from build123d import *

# Parameters (mm, degrees)
SKETCH1_W           = 50
SKETCH1_H           = 15
SKETCH1_R           = 1.5
SKETCH1_R_2         = 5
BOSS_EXTRUDE1_DEPTH = 2.5
SKETCH2_R           = 6
CUT_EXTRUDE1_DEPTH  = 1000
SKETCH5_W           = 20
SKETCH5_H           = 15
BOSS_EXTRUDE2_DEPTH = 15
SKETCH2_5_R         = 6
CUT_EXTRUDE2_DEPTH  = 15
FILLET1_R           = 5
SKETCH6_R           = 1.25
CUT_EXTRUDE3_DEPTH  = 15


with BuildPart() as part:
    # Sketch1 → Boss-Extrude1 (new, symmetric)
    with BuildSketch(Plane(origin=(0, 0, 0), x_dir=(0, 0, -1), z_dir=(1, 0, 0))):
        with Locations((25, 7.5)):
            Rectangle(SKETCH1_W, SKETCH1_H)
        with Locations((10, 7.5)):
            Circle(SKETCH1_R, mode=Mode.SUBTRACT)
        with Locations((17.5, 7.5)):
            Circle(SKETCH1_R_2, mode=Mode.SUBTRACT)
        with Locations((25, 7.5)):
            Circle(SKETCH1_R, mode=Mode.SUBTRACT)
    extrude(amount=BOSS_EXTRUDE1_DEPTH, both=True)

    # Sketch2 → Cut-Extrude1 (cut)
    with BuildSketch(Plane(origin=(0, 15, 0), x_dir=(1, 0, 0), z_dir=(0, 1, 0))):
        with Locations((7.5, 42.75390625)):
            Circle(SKETCH2_R)
    extrude(amount=-CUT_EXTRUDE1_DEPTH, mode=Mode.SUBTRACT)

    # Sketch5 → Boss-Extrude2 (add)
    with BuildSketch(Plane(origin=(0, 15, 0), x_dir=(1, 0, 0), z_dir=(0, 1, 0))):
        with Locations((7.5, 42.5)):
            Rectangle(SKETCH5_W, SKETCH5_H)
    extrude(amount=-BOSS_EXTRUDE2_DEPTH)

    # Sketch2_5 → Cut-Extrude2 (cut)
    with BuildSketch(Plane(origin=(0, 15, 0), x_dir=(1, 0, 0), z_dir=(0, 1, 0))):
        with Locations(Location((7.5, 42.75390625, 0), (0, 0, 270))):
            Circle(SKETCH2_5_R)
    extrude(amount=-CUT_EXTRUDE2_DEPTH, mode=Mode.SUBTRACT)

    # Fillet1
    fillet1_edges = [part.edges().sort_by_distance(p)[0] for p in [
        (17.5, 7.5, -35),
        (17.5, 7.5, -50),
    ]]
    fillet(fillet1_edges, radius=FILLET1_R)

    # Sketch6 → Cut-Extrude3 (cut)
    with BuildSketch(Plane(origin=(17.5, 0, 0), x_dir=(0, 0, -1), z_dir=(1, 0, 0))):
        with Locations((42.5, 7.5)):
            Circle(SKETCH6_R)
    extrude(amount=-CUT_EXTRUDE3_DEPTH, mode=Mode.SUBTRACT)


solid = part.part
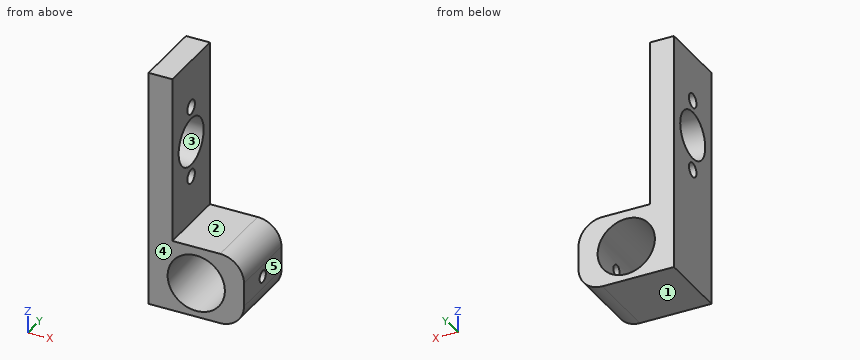
CAD build for the part. Positions are in the model's coordinates, mm. Face numbers are marked on the shaded views. A direction names the side the tool comes from. Give positions to 0.01 mm unless a question says otherwise; leave off trailing zeros. Loops run counter-clockwise (first coordinate to the right, second up) from the corner with the lowest first, then second, coordinate; pieces in that order, holes last. Notation, with made-up numbers: M 31,65.25 L 51,65.25 A13 cw 51,81.25 Z; hole C 24,4 d4. An arc over 180 degrees is marked long. Answer in a Markdown table with one row per item. Add a question column.
Item 1: Band-saw the part on A-A on z = -17.5. Give the cut face in (x, y).
Item 2: Band-saw the part on D-D on z = -42.5. Give the cut face in (x, y).
Item 3: Drop flat-ended pins along their axis: P1, Ø7.5, axis at y = 4, z = -19.5, coming from the +X side; P2, Ø5, axis at x = 9, y = 5.5, coming from the +Z side. Give the stop position or say it passes through.
Item 4: Probe probe 1 along Y at (x, z) = (14.7, -42.5); probe 2 along Z at (x, y) = (7.75, 12.75); probe 3 along X at (y, z) = (1.25, -43). List the from-to ranges inside material, lowest first.
Item 5: Band-saw the part on C-C on x = 7.5. Give the cut face in (y, z).
Item 6: Band-saw the part on B-B on y = 3.75. Give the cut face in (x, z), then the cut area to 3 significant figures.
Item 7: Tool access for the marked faces 1 and 2: list every direction of +Z, -Z, +X, -X, +Y, -Y with a clear straight run to the whole face (end or side of a thin tool).
Item 8: Mould opens along Y. For the marked faces 3, 4 and 5 say: +Y half, -Y half, draft (parallel to the pull), parting line (faces both ways), or undercut.
Reply:
| question | item | result |
|---|---|---|
| 1 | outline | M -2.5,0 L 2.5,0 L 2.5,2.5 L -2.5,2.5 Z; M -2.5,12.5 L 2.5,12.5 L 2.5,15 L -2.5,15 Z |
| 2 | outline | M -2.5,0 L 1.51,0 L 1.51,15 L -2.5,15 Z; M 13.49,0 L 17.5,0 L 17.5,6.25 L 13.49,6.25 Z; M 13.49,8.75 L 17.5,8.75 L 17.5,15 L 13.49,15 Z |
| 3 | P1 | stops at x = 2.5 |
| 3 | P2 | stops at z = -35 |
| 4 | probe 1 | y = 0 to 6.25, 8.75 to 15 |
| 4 | probe 2 | z = -50 to -48.75, -36.76 to -35 |
| 4 | probe 3 | x = -2.5 to 1.51, 13.49 to 17.5 |
| 5 | outline | M 0,-50 L 15,-50 L 15,-48.75 L 0,-48.75 Z; M 0,-36.75 L 15,-36.75 L 15,-35 L 0,-35 Z |
| 6 | outline | M -2.5,-50 L 12.5,-50 A5 ccw 17.5,-45 L 17.5,-40 A5 ccw 12.5,-35 L 2.5,-35 L 2.5,-20.81 L -2.5,-20.81 Z; M -2.5,-14.19 L 2.5,-14.19 L 2.5,0 L -2.5,0 Z; hole C 7.5,-42.75 d12 |
| 6 | area | 318 mm^2 |
| 7 | face 1 | -Z, +X, -X, +Y, -Y |
| 7 | face 2 | +Z, +X, +Y, -Y |
| 8 | face 3 | undercut |
| 8 | face 4 | -Y half |
| 8 | face 5 | draft |
